from build123d import *

# Parameters (mm, degrees)
BOSS_EXTRUDE1_DEPTH = 10
BOSS_EXTRUDE2_DEPTH = 3.5
CUT_EXTRUDE1_REACH  = 40.526
CUT_EXTRUDE2_REACH  = 40.526


with BuildPart() as part:
    # Sketch1 → Boss-Extrude1 (new, symmetric)
    with BuildSketch(Plane.XY):
        Polygon((0, 28), (0, 0), (28, 0), (28, 3.5), (3.5, 3.5), (3.5, 28), align=None)
    extrude(amount=BOSS_EXTRUDE1_DEPTH, both=True)

    # Sketch2 → Boss-Extrude2 (add)
    with BuildSketch(Plane.XY.offset(10)):
        Polygon((3.5, 28), (6, 28), (6, 23), (23, 6), (28, 6), (28, 3.5), (3.5, 3.5), align=None)
    boss_extrude2 = extrude(amount=-BOSS_EXTRUDE2_DEPTH)

    # Mirror1: Boss-Extrude2 across plane
    add(boss_extrude2.mirror(Plane.XY))

    # Sketch3 → Cut-Extrude1 (cut, up to next)
    with BuildSketch(Plane(origin=(0, 3.5, 0), x_dir=(1, 0, 0), z_dir=(0, 1, 0)), mode=Mode.PRIVATE) as cut_extrude1_sk1:
        with BuildLine():
            Line((13, 3), (17, 3))
            ThreePointArc((17, 3), (20, 0), (17, -3))
            Line((17, -3), (13, -3))
            ThreePointArc((13, -3), (10, 0), (13, 3))
        make_face()
    cut_extrude1_tool1 = extrude(cut_extrude1_sk1.sketch, amount=-CUT_EXTRUDE1_REACH, mode=Mode.PRIVATE) & part.part
    add(cut_extrude1_tool1.solids().sort_by_distance((15, 3.5, 0))[0], mode=Mode.SUBTRACT)

    # Sketch4 → Cut-Extrude2 (cut, up to next)
    with BuildSketch(Plane(origin=(3.5, 0, 0), x_dir=(0, 0, -1), z_dir=(1, 0, 0)), mode=Mode.PRIVATE) as cut_extrude2_sk1:
        with BuildLine():
            Line((-3, 13), (-3, 17))
            ThreePointArc((-3, 17), (0, 20), (3, 17))
            Line((3, 17), (3, 13))
            ThreePointArc((3, 13), (0, 10), (-3, 13))
        make_face()
    cut_extrude2_tool1 = extrude(cut_extrude2_sk1.sketch, amount=-CUT_EXTRUDE2_REACH, mode=Mode.PRIVATE) & part.part
    add(cut_extrude2_tool1.solids().sort_by_distance((3.5, 15, 0))[0], mode=Mode.SUBTRACT)


solid = part.part
Model file for the job. Use its own axes, mm. A direction names the side the tool comes from. Round coordinates to 2 decimals unless told otherwise and drop trailing zeros. Order: outer loops, then holes, each group sorted by start corner. A loop starts at its lowest first (then second) coordinate and runs counter-clockwise, first axis right, second up.
(1) Band-saw the part on D-D (y = 24.25). List the corners of the cut face in (x, z).
(2) Pull direction Z, two halves, no side cores. Call faces 5 (the face through (11, 11, 10)), 6 (the face through (10, 10, 6.5)), 7 (the face through (2, 10, 0)), 8 (the face through (10.7, 0, 2.4)): released by +Z, released by -Z, zero draft, split by the parting line, or undercut.
(3) Band-saw the part on B-B (x = 22.5). List the corners of the cut face in (y, z), then the cut area to 3 significant figures.
(4) 3-axis set-ups, long thin cutter, end or side, ignore diameter. For faces 1 (the face through (3.5, 18, 3)), 2 (the face through (20, 2, 0)), 3 (the face through (6, 26, -8)), 4 (the face through (2, 15, 3)): which of +Z, -Z, +X, -X, +Y, -Y reach the whole face in a straight line?
(5) Band-saw the part on C-C (x = 19.5). List the corners of the cut face in (y, z), then the cut area to 3 significant figures.
(6) Pin check, flat tips, straight feed: pin 1 (2 mm diameter, centred on x = 7, z = -3, fed in from +Y); pin 2 (4 mm diameter, centred on y = 9.5, z = -1, fed in from +X); pin 3 (2 mm diameter, centred on x = 19, z = -3, fed in from -Y); pin 4 (1.8 mm diameter, centred on x = 26.5, z = 9, fed in from +Y). Stop position of each tip, or through.
(7) Drill centre lines: line 1 (Z direction, x = 6, y = 15.5); line 2 (X direction, y = 4, z = 5); line 3 (Z direction, x = 2.25, y = 14.5). Where is each one in solid material? Low to high.
(8) Band-saw the part on A-A (y = 14). List the corners of the cut face in (x, z).
Verdict:
1. outline: (0, -10) - (6, -10) - (6, -6.5) - (3.5, -6.5) - (3.5, 6.5) - (6, 6.5) - (6, 10) - (0, 10) - close
2. face 5: released by +Z
2. face 6: undercut
2. face 7: undercut
2. face 8: zero draft
3. outline: (0, -10) - (6.5, -10) - (6.5, -6.5) - (3.5, -6.5) - (3.5, 6.5) - (6.5, 6.5) - (6.5, 10) - (0, 10) - close
3. area: 91.0 mm2
4. face 1: +X, +Y
4. face 2: +Y, -Y
4. face 3: +Z, -Z, +X, +Y
4. face 4: +X, -X
5. outline: (0, -10) - (9.5, -10) - (9.5, -6.5) - (3.5, -6.5) - (3.5, -1.66) - (0, -1.66) - close; (0, 1.66) - (3.5, 1.66) - (3.5, 6.5) - (9.5, 6.5) - (9.5, 10) - (0, 10) - close
5. area: 100 mm2
6. pin 1: stops at y = 3.5
6. pin 2: stops at x = 3.5
6. pin 3: stops at y = 0
6. pin 4: stops at y = 6
7. line 1: z = -10 to -6.5, 6.5 to 10
7. line 2: x = 0 to 3.5
7. line 3: z = -10 to -3, 3 to 10
8. outline: (0, -10) - (15, -10) - (15, -6.5) - (3.5, -6.5) - (3.5, -3) - (0, -3) - close; (0, 3) - (3.5, 3) - (3.5, 6.5) - (15, 6.5) - (15, 10) - (0, 10) - close
